from build123d import *

# Parameters (mm, degrees)
F0_W     = 10
F0_H     = 15
F0_R     = 3
F0_R_2   = 1.6
F1_DEPTH = 2
F3_DEPTH = 15
F2_R     = 2.5
F4_DEPTH = 10.001


with BuildPart() as f1:
    # F0 (on Top) → F1 (new body)
    with BuildSketch(Plane.XY):
        with Locations((5, 7.5)):
            Rectangle(F0_W, F0_H)
        with Locations((5, 4)):
            Circle(F0_R, mode=Mode.SUBTRACT)
        with Locations((5, 12)):
            Circle(F0_R_2, mode=Mode.SUBTRACT)
    extrude(amount=F1_DEPTH)

    # F0 (on Top) → F3 (join)
    with BuildSketch(Plane.XY):
        with Locations((5, 4)):
            Circle(F0_R)
    extrude(amount=F3_DEPTH)

    # F2 (on Right) → F4 (cut, through all)
    with BuildSketch(Plane.YZ):
        with Locations((0, 10.407558)):
            Circle(F2_R)
    extrude(amount=F4_DEPTH, mode=Mode.SUBTRACT)


solid = f1.part
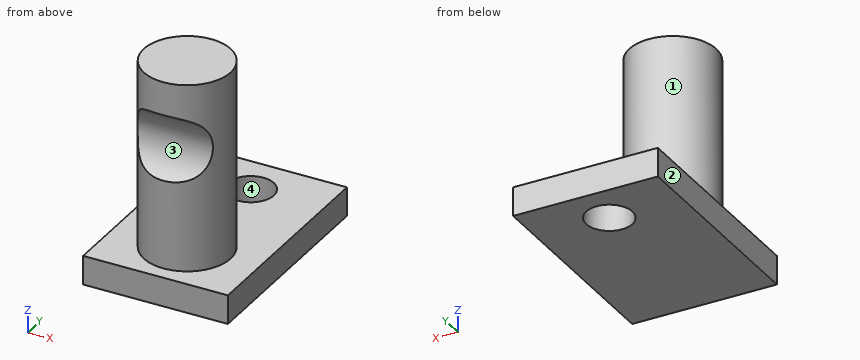
Here's how the part is built. I have some questions about the finished solid (model axes, mm). Face numbers are marked on the shaded views. Coordinates: 2 decimals unless noted, no trailing zeros. Order: outer loops, then holes, each group sorted by start corner. A loop starts at its lowest first (then second) coordinate and runs counter-clockwise, first axis right, second up. Notation, with made-up numbers: M 18.5,-1.75 L 44.5,-1.75 A25 cw 44.5,14.25 Z; hole C 71.25,15.25 d2. An arc over 180 degrees is marked long. Answer as CSV lines item,"result". Start each with the question number.
1. I want a section at A-A, the plane x = 5. Write out the boundary of the cut face in (y, z).
2. I need wall thicknesses on line 1 (Y direction, x = 5, z = 0.95); line 2 (X direction, y = 5.5, z = 3.25); line 3 (Z direction, x = 1.25, y = 1.75). Which ranges of each line are inside material? Lowest first, please. Write a range as [from, to].
3. I want a section at C-C, the plane y = 4. Write out the boundary of the cut face in (x, z), and give its area (3 significant figures).
4. I want a section at D-D, the plane z = 1.5. Write out the boundary of the cut face in (x, y), and give its area (3 significant figures).
5. For pin 1 (2 mm diameter, centred on x = 7, z = 2.5, fed in from -Y); pin 2 (2 mm diameter, centred on x = 7.5, z = 8, fed in from +Y); pin 3 (3 mm diameter, centred on x = 3.5, y = 9.5, fed in from +Z), each with a flat end and sliding along its axis, tell me the tip position at first contact or that it passes through.
6. I want a section at B-B, the plane y = 12. Write out the boundary of the cut face in (x, z).
7. We'd pull the mould along X, two halves only. Please class the marked faces 1, 2, 3 and 4: released by +X, released by -X, zero draft, split by the parting line, or undercut.
Recorded:
1,outline,"M 0,0 L 10.4,0 L 10.4,2 L 7,2 L 7,15 L 1,15 L 1,12.7 A2.5 cw 1,8.12 L 1,2 L 0,2 Z; M 13.6,0 L 15,0 L 15,2 L 13.6,2 Z"
2,line 1,"y = [0, 10.4], [13.6, 15]"
2,line 2,"x = [2.4, 7.6]"
2,line 3,"z = [0, 2]"
3,outline,"M 0,0 L 10,0 L 10,2 L 8,2 L 8,15 L 2,15 L 2,2 L 0,2 Z"
3,area,"98.0 mm2"
4,outline,"M 0,0 L 10,0 L 10,15 L 0,15 Z; hole C 5,12 d3.2"
4,area,"142 mm2"
5,pin 1,"stops at y = 0"
5,pin 2,"stops at y = 6.6"
5,pin 3,"stops at z = 2"
6,outline,"M 0,0 L 3.4,0 L 3.4,2 L 0,2 Z; M 6.6,0 L 10,0 L 10,2 L 6.6,2 Z"
7,face 1,"split by the parting line"
7,face 2,"released by -X"
7,face 3,"zero draft"
7,face 4,"undercut"
